Could you check a few things on this model? Use its own coordinates, in mm. Face numbers are marked on the shaded views. Round coordinates to 2 decimals unless told otherwise and drop trailing zeros. Write each loop counter-clockwise with the first axis right and the second up, starting at its lowest first coordinate (ties: lowest second). Pieces come first, ordered by that corner, then holes. Notation, with made-up numbers: M -10.5,-17 L 31.5,-17 A24 ccw 31.5,-6 Z; hole C -11.5,51 d5. An arc over 180 degrees is marked long. One line per item, written item: value. Start each with the question number.
(1) I want a section at D-D on y = -65. Please give me the cut outline in (x, z), and give its area (3 significant figures).
(2) If I drill on L1, parallel to Z at x = 26, y = -77.5; L2, parallel to Y at x = 115, z = 7.25, over which ranges is the centre line in solid material (lowest first)?
(3) I want a section at C-C on z = 9. Please give me the cut outline in (x, y).
(4) I want a section at B-B on x = 111. Please give me the cut outline in (y, z), and give its area (3 significant figures).
(5) Thinking about a two-plate mould opening in X: for the marked faces 1, 2, 3 and 4, which applies, released by +X, released by -X, zero draft, split by the parting line, or undercut?
(6) I'm going to push flat-ended pins straight in: pin 1 Ø25 at (x, y) = (103, -21.5) entering from +Z; pin 2 Ø8 at (x, z) = (105.5, 19) entering from -Y; pin 3 Ø3 at (x, y) = (150.5, -27.5) entering from +Z. Where does each tip first touch, or does it pass through?
(7) I want a section at A-A on z = 30. Please give me the cut outline in (x, y).
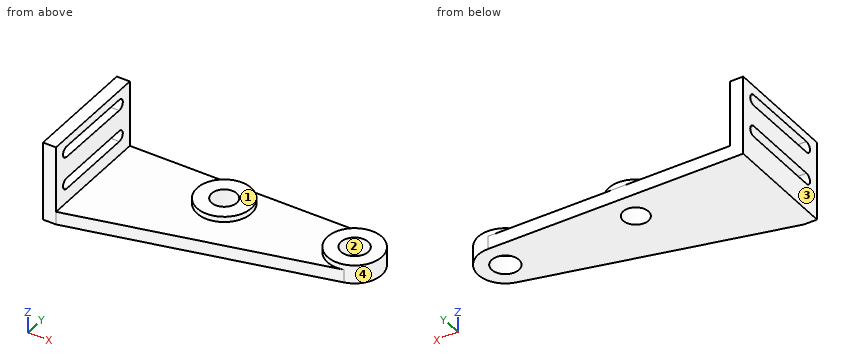
```python
from build123d import *

# Parameters (mm, degrees)
SKETCH1_R            = 25
SKETCH1_R_2          = 11.619106241
SKETCH1_R_3          = 12.5
BOSS_EXTRUDE41_DEPTH = 12
SKETCH1_11_W         = 12
SKETCH1_11_H         = 105
BOSS_EXTRUDE42_DEPTH = 73
BOSS_EXTRUDE43_START = 12
SKETCH1_12_R         = 25
SKETCH1_12_R_2       = 11.619106241
SKETCH1_12_R_3       = 12.5
BOSS_EXTRUDE43_DEPTH = 5
CUT_EXTRUDE1_DEPTH   = 280.030464287


with BuildPart() as part:
    # Sketch1 → Boss-Extrude41 (new body)
    # profile 1 of 3: a face of its own
    with BuildSketch(Plane.XY):
        with BuildLine():
            Line((115, 0), (12, 0))
            Line((12, 0), (12, -105))
            Line((12, -105), (240.911574023, -49.291012588))
            ThreePointArc((240.911574023, -49.291012588), (210.177879676, -27.976968701), (235, 0))
            Line((235, 0), (115, 0))
        make_face()
        with BuildLine():
            ThreePointArc((140, -25), (97.32233047, -42.67766953), (115, 0))
            ThreePointArc((115, 0), (132.67766953, -7.32233047), (140, -25))
        make_face(mode=Mode.SUBTRACT)
    # profile 2 of 3: a face of its own
    with BuildSketch(Plane.XY):
        with Locations((115, -25)):
            Circle(SKETCH1_R)
        with Locations((115, -25)):
            Circle(SKETCH1_R_2, mode=Mode.SUBTRACT)
    # profile 3 of 3: a face of its own
    with BuildSketch(Plane.XY):
        with Locations((235, -25)):
            Circle(SKETCH1_R)
        with Locations((235, -25)):
            Circle(SKETCH1_R_3, mode=Mode.SUBTRACT)
    extrude(amount=BOSS_EXTRUDE41_DEPTH)

    # Sketch1<11> → Boss-Extrude42 (add)
    with BuildSketch(Plane.XY):
        with Locations((6, -52.5)):
            Rectangle(SKETCH1_11_W, SKETCH1_11_H)
    extrude(amount=BOSS_EXTRUDE42_DEPTH)

    # Sketch1<12> → Boss-Extrude43 (add)
    # profile 1 of 2: a face of its own
    with BuildSketch(Plane.XY.offset(BOSS_EXTRUDE43_START)):
        with Locations(Location((115, -25, 0), (0, 0, 90))):
            Circle(SKETCH1_12_R)
        with Locations((115, -25)):
            Circle(SKETCH1_12_R_2, mode=Mode.SUBTRACT)
    # profile 2 of 2: a face of its own
    with BuildSketch(Plane.XY.offset(BOSS_EXTRUDE43_START)):
        with Locations(Location((235, -25, 0), (0, 0, 90))):
            Circle(SKETCH1_12_R)
        with Locations((235, -25)):
            Circle(SKETCH1_12_R_3, mode=Mode.SUBTRACT)
    extrude(amount=BOSS_EXTRUDE43_DEPTH)

    # Sketch2 → Cut-Extrude1 (cut, through all)
    with BuildSketch(Plane(origin=(12, 0, 0), x_dir=(0, 0, -1), z_dir=(1, 0, 0))):
        with BuildLine():
            Line((-54.435034179, -15.03767278), (-55.000141926, -90.03767278))
            ThreePointArc((-55.000141926, -90.03767278), (-60.03767278, -94.999858074), (-64.999858074, -89.96232722))
            Line((-64.999858074, -89.96232722), (-64.434750327, -14.96232722))
            ThreePointArc((-64.434750327, -14.96232722), (-59.397219473, -10.000141926), (-54.435034179, -15.03767278))
        make_face()
        with BuildLine():
            Line((-25, -15), (-25, -90))
            ThreePointArc((-25, -90), (-30, -95), (-35, -90))
            Line((-35, -90), (-35, -15))
            ThreePointArc((-35, -15), (-30, -10), (-25, -15))
        make_face()
    extrude(amount=-CUT_EXTRUDE1_DEPTH, mode=Mode.SUBTRACT)


solid = part.part
```
Found:
1. outline: M 0,0 L 176.36,0 L 176.36,12 L 12,12 L 12,25 L 0,25 Z; M 0,35 L 12,35 L 12,54.81 L 0,54.81 Z; M 0,64.81 L 12,64.81 L 12,73 L 0,73 Z
1. area: 2,610 mm²
2. L1: z = 0 to 12
2. L2: y = -79.93 to -36.62, -13.38 to 0
3. outline: M 0,-105 L 12,-105 L 240.91,-49.29 A25 ccw 235,0 L 0,0 Z; hole C 115,-25 d23.24; hole C 235,-25 d25
4. outline: M -80.91,0 L -35.91,0 L -35.91,17 L -49.68,17 L -49.68,12 L -80.91,12 Z; M -14.09,0 L 0,0 L 0,12 L -0.32,12 L -0.32,17 L -14.09,17 Z
4. area: 847 mm²
5. face 1: zero draft
5. face 2: undercut
5. face 3: released by -X
5. face 4: undercut
6. pin 1: stops at z = 17
6. pin 2: stops at y = -49.26
6. pin 3: stops at z = 12
7. outline: M 0,-105 L 12,-105 L 12,-95 L 0,-95 Z; M 0,-10 L 12,-10 L 12,0 L 0,0 Z
